```python
from build123d import *

# Parameters (mm, degrees)
SKETCH3_W               = 25.4
SKETCH3_H               = 12.7
SKETCH3_W_2             = 22.225
SKETCH3_H_2             = 9.525
BOSS_EXTRUDE1_DEPTH     = 152.4
SKETCH4_R               = 2
CUT_EXTRUDE1_DEPTH      = 1.5875
SKETCH5_R               = 1.500419334
CUT_EXTRUDE2_DEPTH      = 1.5875
CUT_EXTRUDE3_DEPTH      = 154.454683865
CUT_EXTRUDE3_DEPTH_BACK = 2.54
SKETCH7_W               = 20.700000002
SKETCH7_H               = 40.2
CUT_EXTRUDE4_DEPTH      = 154.454683865
M4X0_7_TAPPED_HOLE1_D   = 3.3


with BuildPart() as part:
    # Sketch3 → Boss-Extrude1 (new body)
    with BuildSketch(Plane.XY):
        Rectangle(SKETCH3_W, SKETCH3_H)
        Rectangle(SKETCH3_W_2, SKETCH3_H_2, mode=Mode.SUBTRACT)
    extrude(amount=BOSS_EXTRUDE1_DEPTH)

    # Sketch4 → Cut-Extrude1 (cut)
    with BuildSketch(Plane(origin=(0, 6.35, 0), x_dir=(1, 0, 0), z_dir=(0, 1, 0))):
        with Locations(Location((0, -141.4, 0), (0, 0, 270))):
            Circle(SKETCH4_R)
    extrude(amount=-CUT_EXTRUDE1_DEPTH, mode=Mode.SUBTRACT)

    # Sketch5 → Cut-Extrude2 (cut)
    with BuildSketch(Plane.XZ.offset(6.35)):
        with Locations((-8, 141.4)):
            Circle(SKETCH5_R)
        with Locations((0, 149.4)):
            Circle(SKETCH5_R)
        with Locations((8, 141.4)):
            Circle(SKETCH5_R)
    extrude(amount=-CUT_EXTRUDE2_DEPTH, mode=Mode.SUBTRACT)

    # Sketch6 → Cut-Extrude3 (cut, two sides: drawn at the far end of the back side and taken through both)
    with BuildSketch(Plane.XZ.offset(6.35).offset(-CUT_EXTRUDE3_DEPTH_BACK)):
        Polygon((-5, 469.248822712), (-5, 152.4), (-5, 136.4), (5, 136.4), (5, 152.4), (5, 469.248822712), (5, 1102.946468137), (-5, 1102.946468137), align=None)
    extrude(amount=CUT_EXTRUDE3_DEPTH + CUT_EXTRUDE3_DEPTH_BACK, mode=Mode.SUBTRACT)

    # Sketch7 → Cut-Extrude4 (cut, through all)
    with BuildSketch(Plane.XZ.offset(6.35)):
        with Locations((0, 20.1)):
            Rectangle(SKETCH7_W, SKETCH7_H)
    extrude(amount=-CUT_EXTRUDE4_DEPTH, mode=Mode.SUBTRACT)

    # M4x0.7 Tapped Hole1 (through all)
    with Locations(Plane(origin=(0, -6.35, 0), x_dir=(-1, 0, 0), z_dir=(0, -1, 0))):
        with Locations((-6.35, -50.875), (6.35, -50.875)):
            Hole(M4X0_7_TAPPED_HOLE1_D / 2)


solid = part.part
```
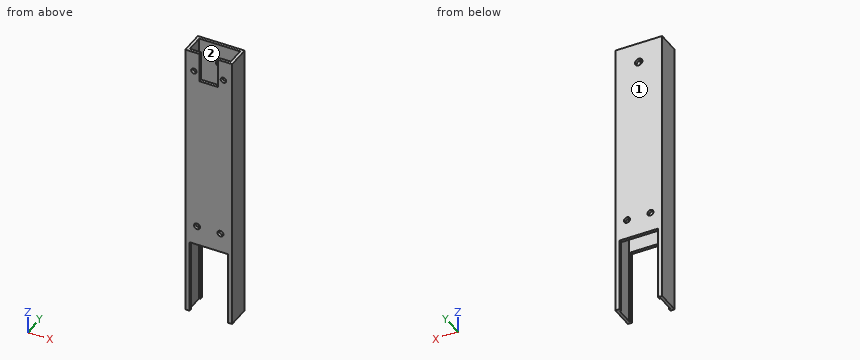
Design review of the part built by this model. Coordinates are the model's own, in mm. Face numbers are marked on the shaded views. Give positions to 0.01 mm unless a question says otherwise; leave off trailing zeros. Write each loop counter-clockwise with the first axis right and the second up, starting at its lowest first coordinate (ties: lowest second). Pieces come first, ordered by that corner, then holes. Notation, with made-up numbers: (3.25, 77) -> (28.25, 77) arc R18 cw to (28.25, 95) -> close; hole circle Ø3 at (74.5, 6.5). An arc over 180 degrees is marked (long way). Answer in a Markdown table with one row per item.
(1) Clearance check with flat-ended pins moving along their axes: pin 1 (2 mm diameter, centred on x = -6.35, z = 50.875, fed in from -Y); pin 2 (1.3 mm diameter, centred on x = -4.5, y = -6, fed in from -Z). State where each tip first meets the part, or that it passes through.
Results:
| item | result |
|---|---|
| pin 1 | through |
| pin 2 | z = 40.2 |
(2) Consider section B-B (y = 1). State the section outline as (x, z) points.
Results:
| item | result |
|---|---|
| outline | (-12.7, 0) -> (-11.11, 0) -> (-11.11, 152.4) -> (-12.7, 152.4) -> close; (11.11, 0) -> (12.7, 0) -> (12.7, 152.4) -> (11.11, 152.4) -> close |
(3) To check wall thickness, follow probe 1 along X at (y, z) = (-5.25, 141.4); probe 2 along Y at (x, z) = (1.25, 101); probe 3 along X at (y, z) = (-1, 14.5). State the ranges of each line that lie inside material, in increasing order.
Results:
| item | result |
|---|---|
| probe 1 | -12.7 to -9.5, -6.5 to -5, 5 to 6.5, 9.5 to 12.7 |
| probe 2 | -6.35 to -4.76, 4.76 to 6.35 |
| probe 3 | -12.7 to -11.11, 11.11 to 12.7 |
(4) Consider section A-A (x = 0). State the section outline as (y, z) points.
Results:
| item | result |
|---|---|
| outline | (-6.35, 40.2) -> (-4.76, 40.2) -> (-4.76, 136.4) -> (-6.35, 136.4) -> close; (4.76, 40.2) -> (6.35, 40.2) -> (6.35, 139.4) -> (4.76, 139.4) -> close; (4.76, 143.4) -> (6.35, 143.4) -> (6.35, 152.4) -> (4.76, 152.4) -> close |
(5) Mouldability with a two-part tool opening along X and no side actions: class the marked faces 1 and 2 as +X half, -X half, draft (parallel to the pull), parting line (faces both ways), or undercut.
Results:
| item | result |
|---|---|
| face 1 | draft |
| face 2 | undercut |
(6) Consider section C-C (z = 103). State the section outline as (x, y) points, then the cut area to 3 significant figures.
Results:
| item | result |
|---|---|
| outline | (-12.7, -6.35) -> (12.7, -6.35) -> (12.7, 6.35) -> (-12.7, 6.35) -> close; hole (-11.11, -4.76) -> (11.11, -4.76) -> (11.11, 4.76) -> (-11.11, 4.76) -> close |
| area | 111 mm2 |
